For this review, take the finished solid that the model builds, in its own axes (mm). Face numbers are marked on the shaded views. A direction names the side the tool comes from. Give positions to 0.01 mm unless a question says otherwise; leave off trailing zeros. Write each loop counter-clockwise with the first axis right and the second up, starting at its lowest first coordinate (ties: lowest second). Pieces come first, ordered by that corner, then holes. Notation, with made-up numbers: (40.5, 26) -> (73.5, 26) arc R25 cw to (73.5, 44) -> close; hole circle Ø8 at (15, 15). An arc over 180 degrees is marked (long way). Answer as CSV lines item,"result".
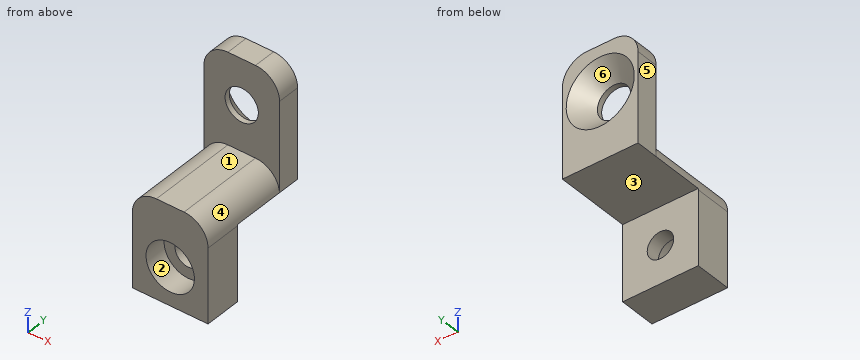
```python
from build123d import *

# Parameters (mm, degrees)
BOSS_EXTRUDE1_DEPTH = 5
FILLET2_R           = 3.175


with BuildPart() as part:
    # Sketch1 → Boss-Extrude1 (new, symmetric)
    with BuildSketch(Plane(origin=(0, 0, 0), x_dir=(0, 0, -1), z_dir=(1, 0, 0))):
        Polygon((-12, 0), (0, 0), (0, -11.87), (13, -11.87), (13, -7), (3, -7), (3, 3), (-12, 3), align=None)
    extrude(amount=BOSS_EXTRUDE1_DEPTH, both=True)

    # Sketch4 → Cut-Revolve1 (revolve, cut)
    with BuildSketch(Plane(origin=(0, 0, 0), x_dir=(0, 0, -1), z_dir=(1, 0, 0)), mode=Mode.PRIVATE) as cut_revolve1_sk:
        Polygon((-6, 3), (-10.5, 3), (-8.2, 0.7), (-8.2, 0), (-6, 0), align=None)
    revolve(cut_revolve1_sk.sketch.rotate(Axis((0, 0, 6), (0, 1, 0)), 180), axis=Axis((0, 0, 6), (0, 1, 0)), mode=Mode.SUBTRACT)

    # Sketch5 → Cut-Revolve2 (revolve, cut)
    with BuildSketch(Plane(origin=(0, 0, 0), x_dir=(0, 0, -1), z_dir=(1, 0, 0))):
        Polygon((8, -11.87), (8, -7), (9.75, -7), (9.75, -8.87), (11.2, -8.87), (11.2, -11.87), align=None)
    revolve(axis=Axis((0, -11.87, -8), (0, 1, 0)), mode=Mode.SUBTRACT)

    # Fillet2
    # the kernel refuses this fillet: 3.175 mm, written as the material it takes off along each edge
    with BuildSketch(Plane(origin=(-5, 0, 0), x_dir=(0, 0, -1), z_dir=(0, -1, 0)), Plane(origin=(5, 0, 0), x_dir=(-1, 0, 0), z_dir=(0, -1, 0))) as fillet2_piece_1:
        with BuildLine():
            CenterArc((FILLET2_R, FILLET2_R), FILLET2_R, 180, 90)
            Line((0, FILLET2_R), (0, 0))
            Line((0, 0), (FILLET2_R, 0))
        make_face()
    extrude(amount=19.8075, mode=Mode.SUBTRACT)
    with BuildSketch(Plane(origin=(-5, 10.9375, 12), x_dir=(0, 0, -1), z_dir=(0, -1, 0)), Plane(origin=(5, 10.9375, 12), x_dir=(-1, 0, 0), z_dir=(0, -1, 0))) as fillet2_piece_2:
        with BuildLine():
            CenterArc((FILLET2_R, FILLET2_R), FILLET2_R, 180, 90)
            Line((0, FILLET2_R), (0, 0))
            Line((0, 0), (FILLET2_R, 0))
        make_face()
    extrude(amount=18.875, mode=Mode.SUBTRACT)


solid = part.part
```
Q1. For the marked faces 1, 2 and 3, list the 3-axis set-ups (+Z, -Z, +X, -X, +Y, -Y) from which the entire face can be reached by the end or side of a thin tool; tool diameter is ignored.
Answer block:
face 1,"+Z, +X, -X, -Y"
face 2,"-Y"
face 3,"-Z, +X, -X, +Y"
Q2. Add section A-A (x = 0). Write out the cut boundary in (y, z).
Answer block:
outline,"(-11.87, -13) -> (-7, -13) -> (-7, -9.75) -> (-8.87, -9.75) -> (-8.87, -11.2) -> (-11.87, -11.2) -> close; (-11.87, -4.8) -> (-8.87, -4.8) -> (-8.87, -6.25) -> (-7, -6.25) -> (-7, -3) -> (3, -3) -> (3, 1.5) -> (0.7, 3.8) -> (0, 3.8) -> (0, 0) -> (-11.87, 0) -> close; (0, 8.2) -> (0.7, 8.2) -> (3, 10.5) -> (3, 12) -> (0, 12) -> close"
Q3. Add section C-C (y = 1.75). Write out the cut boundary in (x, z) (3 decimals).
Answer block:
outline,"(-5, -3) -> (5, -3) -> (5, 8.825) arc R3.175 ccw to (1.825, 12) -> (-1.825, 12) arc R3.175 ccw to (-5, 8.825) -> close; hole circle Ø6.5 at (0, 6)"
Q4. Add section D-D (z = 6). Write out the cut boundary in (x, y), plus the area to 3 significant figures.
Answer block:
outline,"(-5, 0) -> (-2.2, 0) -> (-2.2, 0.7) -> (-4.5, 3) -> (-5, 3) -> close; (2.2, 0) -> (5, 0) -> (5, 3) -> (4.5, 3) -> (2.2, 0.7) -> close"
area,"11.5 mm2"
Q5. To check wall thickness, follow probe 1 along X at (y, z) = (-11, -8); probe 2 along X at (y, z) = (-7.7, -8); probe 3 along Y at (x, z) = (-4, 3). State the ranges of each line that lie inside material, in increasing order. Write a range as [from, to].
Answer block:
probe 1,"x = [-5, -3.2], [3.2, 5]"
probe 2,"x = [-5, -1.75], [1.75, 5]"
probe 3,"y = [0, 3]"
Q6. Draft analysis for pull direction X (two halves, no side actions). For the marked faces 4, 5 and 6, state which applies: released by +X, released by -X, zero draft, split by the parting line, or undercut.
Answer block:
face 4,"released by +X"
face 5,"released by -X"
face 6,"undercut"
Q7. Add section B-B (z = -8). Write out the cut boundary in (x, y).
Answer block:
outline,"(-5, -11.87) -> (-3.2, -11.87) -> (-3.2, -8.87) -> (-1.75, -8.87) -> (-1.75, -7) -> (-5, -7) -> close; (1.75, -8.87) -> (3.2, -8.87) -> (3.2, -11.87) -> (5, -11.87) -> (5, -7) -> (1.75, -7) -> close"
Q8. Clearance check with flat-ended pins moving along their axes: pin 1 (4 mm diameter, centred on x = -1, z = -8.5, fed in from +Y); pin 2 (5.5 mm diameter, centred on x = 0, z = -8, fed in from -Y); pin 3 (5 mm diameter, centred on x = 0, z = 6, fed in from +Y). State where each tip first meets the part, or that it passes through.
Answer block:
pin 1,"stops at y = -7"
pin 2,"stops at y = -8.87"
pin 3,"stops at y = 1"
